Read the model definition and answer for the solid it produces. Units are mm, in the model's axes. A direction names the side the tool comes from. Coordinates: 2 decimals unless noted, no trailing zeros. Write each loop counter-clockwise with the first axis right and the second up, starting at its lowest first coordinate (ties: lowest second). Pieces come first, ordered by that corner, then holes.
(1) Section A-A on z = 0.8 is taken. Write down the section's boundary in (x, y).
(2) Section B-B on x = 3.5 is taken. Write down the section's boundary in (y, z), then the cut area to 3 significant figures.
(3) Given pin 1 (0.8 mm diameter, centred on x = -9, y = 33.5, fed in from +Z), flat-ended and moving along its own axis, determine where the tip first touches the part or whether it passes through.
(4) Find the intervals of material crossed by probe 1 along Y at (x, z) = (-15, 0.7); probe 2 along Y at (x, z) = (0, 0.4); probe 3 along Y at (x, z) = (9, 0.95), in increasing order.
(5) Which of the six approach directions +Z, -Z, +X, -X, +Y, -Y give full straight-line access (tool end or side, diameter ignored) to faces 1 (the flat face through (0, 0, 0)), 2 (the flat face through (0, -34, 0.5)), 3 (the flat face through (0, 34, 0.5))?
from build123d import *

# Parameters (mm, degrees)
F0_W     = 70
F0_H     = 65
F0_R     = 0.5
F1_DEPTH = 1
F0_H_2   = 2.5
F2_DEPTH = 0.5


with BuildPart() as f1:
    # F0 (on Top) → F1 (new body)
    with BuildSketch(Plane.XY):
        Rectangle(F0_W, F0_H)
        with Locations((-15, -10)):
            Circle(F0_R, mode=Mode.SUBTRACT)
        with Locations((0, -10)):
            Circle(F0_R, mode=Mode.SUBTRACT)
        with Locations((15, -10)):
            Circle(F0_R, mode=Mode.SUBTRACT)
        with Locations((-15, 10)):
            Circle(F0_R, mode=Mode.SUBTRACT)
        with Locations((0, 10)):
            Circle(F0_R, mode=Mode.SUBTRACT)
        with Locations((15, 10)):
            Circle(F0_R, mode=Mode.SUBTRACT)
    extrude(amount=F1_DEPTH)

    # F0 (on Top) → F2 (join)
    with BuildSketch(Plane.XY):
        Rectangle(F0_W, F0_H)
        with Locations((-15, -10)):
            Circle(F0_R, mode=Mode.SUBTRACT)
        with Locations((0, -10)):
            Circle(F0_R, mode=Mode.SUBTRACT)
        with Locations((15, -10)):
            Circle(F0_R, mode=Mode.SUBTRACT)
        with Locations((-15, 10)):
            Circle(F0_R, mode=Mode.SUBTRACT)
        with Locations((0, 10)):
            Circle(F0_R, mode=Mode.SUBTRACT)
        with Locations((15, 10)):
            Circle(F0_R, mode=Mode.SUBTRACT)
        with Locations((0, 33.75)):
            Rectangle(F0_W, F0_H_2)
        with Locations((0, -33.75)):
            Rectangle(F0_W, F0_H_2)
    extrude(amount=F2_DEPTH)


solid = f1.part
Response:
1. outline: (-35, -32.5) - (35, -32.5) - (35, 32.5) - (-35, 32.5) - close; hole circle Ø1 at (-15, -10); hole circle Ø1 at (-15, 10); hole circle Ø1 at (0, -10); hole circle Ø1 at (0, 10); hole circle Ø1 at (15, -10); hole circle Ø1 at (15, 10)
2. outline: (-35, 0) - (35, 0) - (35, 0.5) - (32.5, 0.5) - (32.5, 1) - (-32.5, 1) - (-32.5, 0.5) - (-35, 0.5) - close
2. area: 67.5 mm2
3. pin 1: stops at z = 0.5
4. probe 1: y = -32.5 to -10.5, -9.5 to 9.5, 10.5 to 32.5
4. probe 2: y = -35 to -10.5, -9.5 to 9.5, 10.5 to 35
4. probe 3: y = -32.5 to 32.5
5. face 1: -Z, +X, -X, +Y, -Y
5. face 2: +Z, +X, -X, -Y
5. face 3: +Z, +X, -X, +Y
